Geometry: see drawing. Coordinates: mm, zero at the bounding-box minimum. Coordinates: 2 decimals unless noted, no trailing zeros. Loops run counter-clockwise (first coordinate to the right, second up) from the corner with the lowest first, then second, coordinate; pieces in that order, holes last. Notation, with made-up numbers: (75.5, -19.5) -> (104.5, -19.5) arc R15 cw to (104.5, 5.5) -> close; hole circle Ø6 at (76, 42). An arc over 180 degrees is marked (long way). Answer as a JSON object with one key per item and string values.
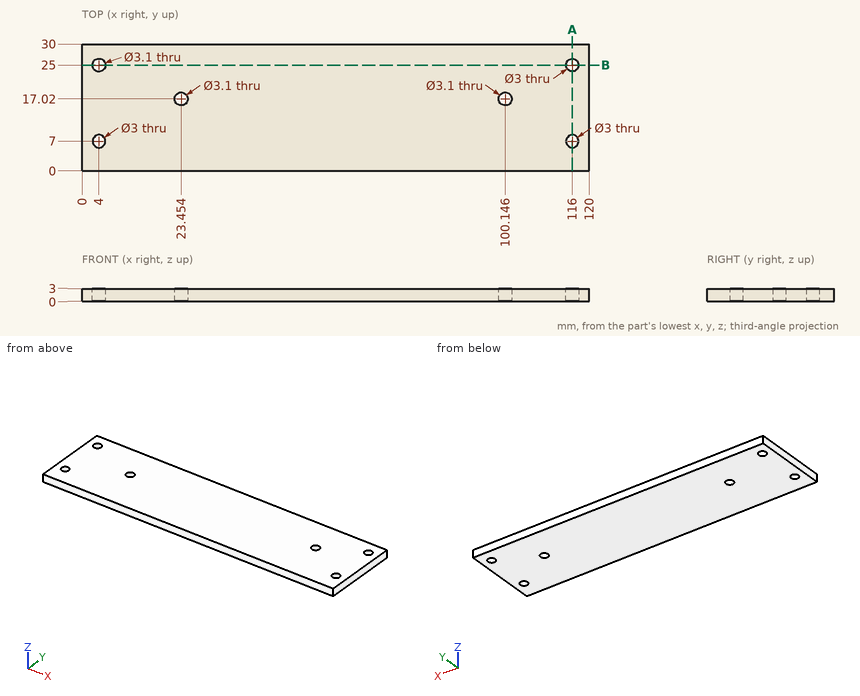
1. Line query: line 1 along Y through (x, z) = (116, 1.3); line 2 along Y through (x, z) = (101, 2.95); line 3 along Y through (x, z) = (100.5, 1.7). Output: solid intervals per line, ascending.
Reply:
{"line 1": "y = 0 to 5.5, 8.5 to 23.5, 26.5 to 30", "line 2": "y = 0 to 15.73, 18.31 to 30", "line 3": "y = 0 to 15.51, 18.53 to 30"}
2. Section query A-A (x = 116). Return loops of the section in (y, z), plus the area to 3 significant figures.
Reply:
{"outline": "(0, 0) -> (5.5, 0) -> (5.5, 3) -> (0, 3) -> close; (8.5, 0) -> (23.5, 0) -> (23.5, 3) -> (8.5, 3) -> close; (26.5, 0) -> (30, 0) -> (30, 3) -> (26.5, 3) -> close", "area": "72.0 mm2"}
3. Section query B-B (y = 25). Return loops of the section in (x, z).
Reply:
{"outline": "(0, 0) -> (2.45, 0) -> (2.45, 3) -> (0, 3) -> close; (5.55, 0) -> (114.5, 0) -> (114.5, 3) -> (5.55, 3) -> close; (117.5, 0) -> (120, 0) -> (120, 3) -> (117.5, 3) -> close"}
